Geometry check sheet. Reference: the model listing, model coordinates, mm. A direction names the side the tool comes from. Round coordinates to 2 decimals unless told otherwise and drop trailing zeros. Order: outer loops, then holes, each group sorted by start corner. A loop starts at its lowest first (then second) coordinate and runs counter-clockwise, first axis right, second up.
(1) Cross-section at D-D on z = 113.5. Enter the section's corners in (x, y).
(2) Cross-section at B-B on y = 0. Enter the section's corners in (x, z), and give its area (3 significant figures).
(3) Set-up check for faces 1 (the face through (4.38, 8.43, 3.45)), 2 (the face through (2.5, 8, 120)), 3 (the face through (-1.302, -9.915, 78.807)): record each of +Z, -Z, +X, -X, +Y, -Y from which the full face is reachable in a straight line by a thin tool's end or side.
(4) Draft check along X on faces 4 (the face through (-0.1, 10.2, 30)), 5 (the face through (0.371, -9.166, 129.826)), 6 (the face through (0, 9, 110)). Enter one of: pulls with the +X half, pulls with the -X half, needs draft (parallel to the pull), parting line crosses it, or undercut.
(5) Gauge pin test, flat ends, axial feed: P1, Ø8, axis at y = -0.5, z = 21, coming from the -X side; P2, Ø12, axis at y = 8, z = 44.5, coming from the +X side; P3, Ø0.8, axis at y = 8, z = 121.5, coming from the -X side; P4, Ø5, axis at x = 2.5, z = 67.5, coming from the +Y side. Record the tip position at first contact, or that the pin passes through.
(6) Cross-section at A-A on x = 0. Enter the section's corners in (y, z), and give its area (3 significant figures).
(7) Thickness scan on L1, parallel to Z at x = 1.5, y = 9; L2, parallel to Z at x = 5.5, y = -6.25; L3, parallel to Z at x = 10.25, y = 6.5. Record the ranges inside material, lowest first.
(8) Cross-section at C-C on z = 62.5. Enter the section's corners in (x, y).
Autodesk Inventor part; units mm, degrees
ref_plane "YZ Plane" through (0, 0, 0) normal (1, 0, 0) x (0, 1, 0)
ref_plane "XZ Plane" through (0, 0, 0) normal (0, 1, 0) x (-1, 0, 0)
ref_plane "XY Plane" through (0, 0, 0) normal (0, 0, 1) x (1, 0, 0)
sketch "Sketch1" plane through (0, 0, 0) normal (0, 0, 1) x (1, 0, 0)
  circle A0 centre (0, 0) radius 9.5
  dimension "d0" = 19
extrude "Extrusion1" add sketch "Sketch1" along normal blind 7
sketch "Sketch2" plane through (0, 0, 7) normal (0, 0, 1) x (1, 0, 0)
  circle A0 centre (0, 0) radius 6.5
  dimension "d3" = 13
extrude "Extrusion2" add sketch "Sketch2" along normal blind 6
sketch "Sketch3" plane through (0, 0, 13) normal (0, 0, 1) x (1, 0, 0)
  circle A0 centre (0, 0) radius 9.5
  dimension "d6" = 19
extrude "Extrusion3" add sketch "Sketch3" along normal blind 7
sketch "Sketch4" plane through (0, 0, 20) normal (0, 0, 1) x (1, 0, 0)
  circle A0 centre (0, 0) radius 12.5
  dimension "d9" = 25
extrude "Extrusion4" add sketch "Sketch4" along normal blind 10
sketch "Sketch5" plane through (0, 0, 30) normal (0, 0, 1) x (1, 0, 0)
  circle A0 centre (0, 0) radius 10
  dimension "d12" = 20
extrude "Extrusion5" add sketch "Sketch5" along normal blind 100
chamfer "Chamfer1" distance 1 angle 45 1 edges at (-10, 0, 130)
sketch "Sketch6" plane through (0, 0, 130) normal (0, 0, 1) x (1, 0, 0)
  line L0 (-2.5, 12) -> (2.5, 12)
  line L1 (2.5, 12) -> (2.5, 7)
  line L2 (2.5, 7) -> (-2.5, 7)
  line L3 (-2.5, 7) -> (-2.5, 12)
  point P0 (0, 0)
  point P1 (0, 7)
  dimension "d18" = 5
  dimension "d19" = 5
  dimension "d20" = 7
extrude "Extrusion6" cut sketch "Sketch6" against normal blind 20
properties part number "shaft"
Found:
1. outline: (-2.5, 7) - (-2.5, 9.68) arc R10 ccw (long way) to (2.5, 9.68) - (2.5, 7) - close
2. outline: (-12.5, 20) - (-9.5, 20) - (-9.5, 13) - (-6.5, 13) - (-6.5, 7) - (-9.5, 7) - (-9.5, 0) - (9.5, 0) - (9.5, 7) - (6.5, 7) - (6.5, 13) - (9.5, 13) - (9.5, 20) - (12.5, 20) - (12.5, 30) - (10, 30) - (10, 129) - (9, 130) - (-9, 130) - (-10, 129) - (-10, 30) - (-12.5, 30) - close
2. area: 2,590 mm2
3. face 1: -Z
3. face 2: +Z, +Y
3. face 3: +Z
4. face 4: needs draft
4. face 5: parting line crosses it
4. face 6: undercut
5. P1: stops at x = -12.5
5. P2: stops at x = 9.8
5. P3: stops at x = -6.5
5. P4: stops at y = 10
6. outline: (-12.5, 20) - (-9.5, 20) - (-9.5, 13) - (-6.5, 13) - (-6.5, 7) - (-9.5, 7) - (-9.5, 0) - (9.5, 0) - (9.5, 7) - (6.5, 7) - (6.5, 13) - (9.5, 13) - (9.5, 20) - (12.5, 20) - (12.5, 30) - (10, 30) - (10, 110) - (7, 110) - (7, 130) - (-9, 130) - (-10, 129) - (-10, 30) - (-12.5, 30) - close
6. area: 2,530 mm2
7. L1: z = 0 to 7, 13 to 110
7. L2: z = 0 to 7, 13 to 130
7. L3: z = 20 to 30
8. outline: circle Ø20 at (0, 0)
